The drawing under review shows one solid part. Ordinate dimensions are in mm from its lowest x, y, z. A direction names the side the tool comes from. Coordinates: 2 decimals unless noted, no trailing zeros. Order: outer loops, then holes, each group sorted by start corner. A loop starts at its lowest first (then second) coordinate and runs counter-clockwise, first axis right, second up. Notation, with made-up numbers: (-14.5, 66) -> (40.5, 66) arc R36 cw to (40.5, 103) -> close; hole circle Ø5 at (-11.75, 56). An arc over 180 degrees is marked (long way). Use one line per item in the form item = value.
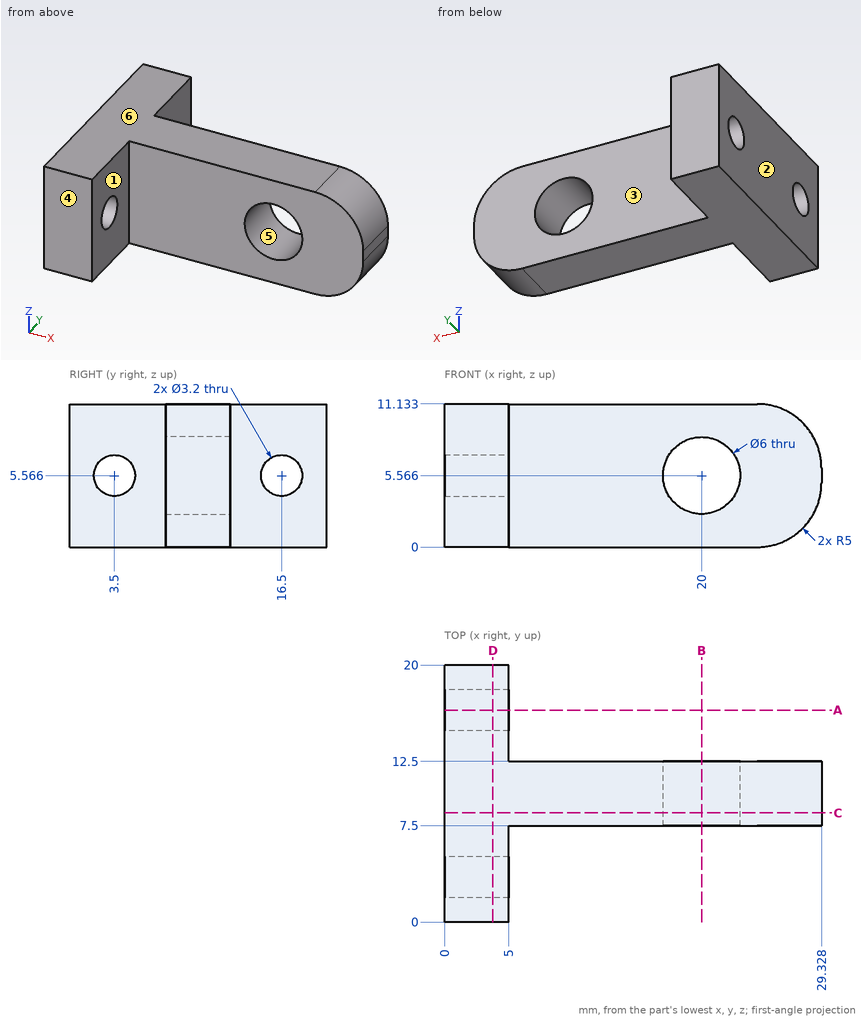
Item 1: Draft analysis for pull direction Z (two halves, no side actions). For the marked faces 4, 5 and 6, state which applies: released by +Z, released by -Z, zero draft, split by the parting line, or undercut.
Results found:
face_4 = zero draft
face_5 = undercut
face_6 = released by +Z
Item 2: To check wall thickness, follow L1, parallel to Z at x = 1.8, y = 3.5; L2, parallel to Y at x = 4, z = 6; L3, parallel to Y at x = 19.25, z = 2.5. State the ranges of each line that lie inside material, in increasing order. Write a range as from..to.
Results found:
L1 = 0..3.97, 7.17..11.13
L2 = 0..1.96, 5.04..14.96, 18.04..20
L3 = 7.5..12.5
Item 3: Tool access review of the marked faces 1, 2 and 3: name each direction out of +Z, -Z, +X, -X, +Y, -Y from which nothing blocks a thin tool from reaching the whole face with its end or side.
Results found:
face_1 = +Z, -Z, +X, -Y
face_2 = +Z, -Z, -X, +Y, -Y
face_3 = +Z, -Z, +X, +Y
Item 4: We need section C-C (y = 8.5). Write out the cut boundary in (x, z).
Results found:
outline = (0, 0) -> (24.33, 0) arc R5 ccw to (29.33, 5) -> (29.33, 6.13) arc R5 ccw to (24.33, 11.13) -> (0, 11.13) -> close; hole circle Ø6 at (20, 5.57)
Item 5: We need section B-B (x = 20). Write out the cut boundary in (y, z).
Results found:
outline = (7.5, 0) -> (12.5, 0) -> (12.5, 2.57) -> (7.5, 2.57) -> close; (7.5, 8.57) -> (12.5, 8.57) -> (12.5, 11.13) -> (7.5, 11.13) -> close
Item 6: We need section D-D (x = 3.75). Write out the cut boundary in (y, z).
Results found:
outline = (0, 0) -> (20, 0) -> (20, 11.13) -> (0, 11.13) -> close; hole circle Ø3.2 at (3.5, 5.57); hole circle Ø3.2 at (16.5, 5.57)
Item 7: Clearance check with flat-ended pins moving along their axes: pin 1 (5 mm diameter, centred on y = 16.5, z = 5.57, fed in from +X); pin 2 (5.5 mm diameter, centred on x = 22.5, z = 3, fed in from +Y); pin 3 (5 mm diameter, centred on x = 21, z = 2, fed in from -Y). State where each tip first meets the part, or that it passes through.
Results found:
pin_1 = 5
pin_2 = 12.5
pin_3 = 7.5
Item 8: We need section A-A (y = 16.5). Write out the cut boundary in (x, z).
Results found:
outline = (0, 0) -> (5, 0) -> (5, 3.97) -> (0, 3.97) -> close; (0, 7.17) -> (5, 7.17) -> (5, 11.13) -> (0, 11.13) -> close
